Input: part model. Units: mm. Frame: model coordinates. A direction names the side the tool comes from. Coordinates: 2 decimals unless noted, no trailing zeros. Write each loop counter-clockwise with the first axis right and the second up, starting at its lowest first coordinate (ties: lowest second). Pieces come first, ordered by that corner, then holes. Notation, with made-up numbers: M -21.5,51.5 L 17.5,51.5 A29 cw 17.5,76.5 Z; hole C 67,63 d1. An arc over 180 degrees is marked long. Use one line per item in the form item = value.
from build123d import *

# Parameters (mm, degrees)
GUIDE_AND_SOLID_STOPS_DEPTH  = 13.6
SKETCH_3_W                   = 8.4
SKETCH_3_H                   = 14
NUT_TONGUE_CHANNEL_DEPTH     = 2.8
SKETCH_4_W                   = 6.25
SKETCH_4_H                   = 5.2
LOWER_YOKE_RELIEF_DEPTH      = 3
SKETCH_5_W                   = 3.7
SKETCH_5_H                   = 3
LOWER_INWARD_STOP_DEPTH      = 3.8
SKETCH_7_W                   = 3.7
SKETCH_7_H                   = 3
EXTRUDE_2_DEPTH              = 3.8
REMOVE_LOWER_TAIL_DEPTH      = 62.002151601
REMOVE_LOWER_TAIL_DEPTH_BACK = 62.002151601
SKETCH_8_W                   = 17
SKETCH_8_H                   = 17


with BuildPart() as part:
    # 草图1 → Guide_and_solid_stops (new body)
    with BuildSketch(Plane.XY):
        Polygon((10.2, 0), (16.95, 0), (16.95, 54), (11.2, 54), (11.2, 57), (4.7, 57), (4.7, 53), (10.2, 53), (10.2, 51.5), (10.95, 51.5), (10.95, 38), (10.2, 38), (10.2, 36), (4.7, 36), (4.7, 32), (10.2, 32), align=None)
    extrude(amount=GUIDE_AND_SOLID_STOPS_DEPTH)

    # 草图3 → Nut_tongue_channel (cut, symmetric)
    with BuildSketch(Plane.XY.offset(6.8)):
        with Locations((11.2, 44.5)):
            Rectangle(SKETCH_3_W, SKETCH_3_H)
    extrude(amount=NUT_TONGUE_CHANNEL_DEPTH, both=True, mode=Mode.SUBTRACT)

    # 草图4 → Lower_yoke_relief (cut, symmetric)
    with BuildSketch(Plane.XY.offset(6.8)):
        with Locations((7.125, 33.6)):
            Rectangle(SKETCH_4_W, SKETCH_4_H)
    extrude(amount=LOWER_YOKE_RELIEF_DEPTH, both=True, mode=Mode.SUBTRACT)

    # 草图5 → Lower_inward_stop (add)
    with BuildSketch(Plane.XY):
        with Locations((9.35, 16.5)):
            Rectangle(SKETCH_5_W, SKETCH_5_H)
    extrude(amount=LOWER_INWARD_STOP_DEPTH)

    # 草图7 → 凸台-拉伸2 (add)
    with BuildSketch(Plane.XY.offset(9.8)):
        with Locations((9.35, 16.5)):
            Rectangle(SKETCH_7_W, SKETCH_7_H)
    extrude(amount=EXTRUDE_2_DEPTH)

    # 草图8 → Remove_lower_tail (cut, two sides: drawn at the far end of the back side and taken through both)
    with BuildSketch(Plane.XY.offset(-REMOVE_LOWER_TAIL_DEPTH_BACK)):
        with Locations((11.5, 6.5)):
            Rectangle(SKETCH_8_W, SKETCH_8_H)
    extrude(amount=REMOVE_LOWER_TAIL_DEPTH + REMOVE_LOWER_TAIL_DEPTH_BACK, mode=Mode.SUBTRACT)


solid = part.part
(1) Section query B-B on x = 8. Return the cut outline in (y, z), plus the area to 3 significant figures.
Computed:
outline = M 15,0 L 18,0 L 18,3.8 L 15,3.8 Z; M 15,9.8 L 18,9.8 L 18,13.6 L 15,13.6 Z; M 32,0 L 36,0 L 36,3.8 L 32,3.8 Z; M 32,9.8 L 36,9.8 L 36,13.6 L 32,13.6 Z; M 53,0 L 57,0 L 57,13.6 L 53,13.6 Z
area = 108 mm^2
(2) Section query A-A on x = 6.25. Return the cut outline in (y, z).
Computed:
outline = M 32,0 L 36,0 L 36,3.8 L 32,3.8 Z; M 32,9.8 L 36,9.8 L 36,13.6 L 32,13.6 Z; M 53,0 L 57,0 L 57,13.6 L 53,13.6 Z
(3) Pull-direction query (Y, two-part tool) for faces 1 (the flat face through (9, 18, 12)), 2 (the flat face through (9, 17, 9.8)), 3 (the flat face through (7, 32, 2)), 4 (the flat face through (14, 54, 7)); classes: pulls with the +Y half, pulls with the -Y half, needs draft (parallel to the pull), parting line crosses it, or undercut.
Computed:
face_1 = undercut
face_2 = needs draft
face_3 = undercut
face_4 = pulls with the +Y half
(4) Line query: probe 1 along Y at (x, z) = (10.25, 10.75); probe 2 along X at (y, z) = (24, 4); probe 3 along Y at (x, z) = (10, 8). Output: solid intervals per line, ascending.
Computed:
probe_1 = 15 to 38, 51.5 to 57
probe_2 = 10.2 to 16.95
probe_3 = 53 to 57
(5) Section query C-C on z = 2.25. Return the cut outline in (x, y).
Computed:
outline = M 4.7,32 L 10.2,32 L 10.2,18 L 7.5,18 L 7.5,15 L 16.95,15 L 16.95,54 L 11.2,54 L 11.2,57 L 4.7,57 L 4.7,53 L 10.2,53 L 10.2,51.5 L 10.95,51.5 L 10.95,38 L 10.2,38 L 10.2,36 L 4.7,36 Z
(6) Set-up query: faces 5 (the flat face through (13, 45, 4)), 6 (the flat face through (13, 36, 13.6)), 7 (the flat face through (10.95, 45, 2)), 8 (the flat face through (7.5, 16, 12)). Return all of +Z, -Z, +X, -X, +Y, -Y with unobstructed straight access to the full face (end or side cutting, diameter ignored); none if empty.
Computed:
face_5 = -X
face_6 = +Z, +X, -X, +Y, -Y
face_7 = +Z, -Z, -X
face_8 = +Z, -Z, -X, -Y
(7) First-contact query: pin 1 Ø4.5 at (y, z) = (45, 7.5) entering from -X; pin 2 Ø4 at (y, z) = (22.5, 4) entering from -X; pin 3 Ø4.5 at (x, z) = (13.5, 6.5) entering from +Y. Flat tips, straight axial feed; report the tip coordinate or a pass-through.
Computed:
pin_1 = 10.95
pin_2 = 10.2
pin_3 = 54
(8) Section query D-D on y = 48. Return the cut outline in (x, z), plus the area to 3 significant figures.
Computed:
outline = M 10.95,0 L 16.95,0 L 16.95,13.6 L 10.95,13.6 L 10.95,9.6 L 15.4,9.6 L 15.4,4 L 10.95,4 Z
area = 56.7 mm^2
